Verification items for the finished model (mm, model axes). A direction names the side the tool comes from. Round coordinates to 2 decimals unless told otherwise and drop trailing zeros. Write each loop counter-clockwise with the first axis right and the second up, starting at its lowest first coordinate (ties: lowest second). Pieces come first, ordered by that corner, then holes. Notation, with made-up numbers: M -13.5,-27 L -3.5,-27 A20 cw -3.5,7 Z; hole C 45.5,-27 d6. An arc over 180 degrees is marked long. One line per question, with ' | ' between items. Start each with the question number.
Q1. Cross-section at C-C (y = -2.5). Record the boundary of the cut face in (x, z) (3 decimals).
Q2. Cross-section at B-B (x = -62). Record the boundary of the cut face in (y, z) (3 decimals).
Q3. Tool access check on faces 1 (the face through (92.5, -51.5, -3.9)), 2 (the face through (-99.48, -1, -6)). Record the directions out of +Z, -Z, +X, -X, +Y, -Y that give a thin tool (end or side, any length) a straight path to the whole face; none if there is none.
Q4. Release check for a two-part mould opening along Y. For faces 3 (the face through (94.06, 52.77, -0.74)), 4 (the face through (1, -58.38, -6)), 5 (the face through (-96.172, 55.243, -5.916)) record: released by +Y, released by -Y, zero draft, split by the parting line, or undercut.
Q5. Cross-section at A-A (z = -4). Record the boundary of the cut face in (x, y).
Q6. Thickness scan on line 1 along X through (y, z) = (2.5, -4.25); line 2 along Y through (x, z) = (-22, -3.75); line 3 along Z through (x, y) = (26.5, -16). Record the ranges inside material, lowest first. Write a range as from..to.
Autodesk Inventor part; units mm, degrees
ref_plane "YZ Plane" through (0, 0, 0) normal (1, 0, 0) x (0, 1, 0)
ref_plane "XZ Plane" through (0, 0, 0) normal (0, 1, 0) x (-1, 0, 0)
ref_plane "XY Plane" through (0, 0, 0) normal (0, 0, 1) x (1, 0, 0)
sketch "Sketch1" plane through (0, 0, 0) normal (0, 0, 1) x (1, 0, 0)
  line L0 (77.5, 43.5) -> (77.5, -43.5)
  line L1 (77.5, -43.5) -> (-77.5, -43.5)
  line L2 (-77.5, -43.5) -> (-77.5, 43.5)
  line L3 (-77.5, 43.5) -> (77.5, 43.5)
  line L4 (85.48, 55.38) -> (-85.48, 55.38)
  arc A0 (-85.48, 55.38) -> (-96.48, 44.38) centre (-85.48, 44.38) ccw
  line L5 (-96.48, 44.38) -> (-96.48, -44.38)
  arc A1 (-96.48, -44.38) -> (-85.48, -55.38) centre (-85.48, -44.38) ccw
  line L6 (-85.48, -55.38) -> (85.48, -55.38)
  arc A2 (85.48, -55.38) -> (96.48, -44.38) centre (85.48, -44.38) ccw
  line L7 (96.48, -44.38) -> (96.48, 44.38)
  arc A3 (96.48, 44.38) -> (85.48, 55.38) centre (85.48, 44.38) ccw
  line L8 (-88.48, 58.38) -> (88.48, 58.38)
  line L9 (99.48, 47.38) -> (99.48, -47.38)
  line L10 (88.48, -58.38) -> (-88.48, -58.38)
  line L11 (-99.48, -47.38) -> (-99.48, 47.38)
  arc A4 (-88.48, 58.38) -> (-99.48, 47.38) centre (-88.48, 47.38) ccw
  arc A5 (99.48, 47.38) -> (88.48, 58.38) centre (88.48, 47.38) ccw
  arc A6 (88.48, -58.38) -> (99.48, -47.38) centre (88.48, -47.38) ccw
  arc A7 (-99.48, -47.38) -> (-88.48, -58.38) centre (-88.48, -47.38) ccw
  point P0 (0, 0)
  dimension "d0" = 3
  dimension "d1" = 3
  dimension "d2" = 3
  dimension "d3" = 3
  dimension "d4" = 11
  dimension "d5" = 11
extrude "Extrusion1" add sketch "Sketch1" against normal blind 12 contours L0 L1 L2 L3 | A3 L7 A2 L6 A1 L5 A0 L4 | L8 A5 L9 A6 L10 A7 L11 A4
sketch "Sketch2" plane through (0, 0, 0) normal (0, 0, 1) x (1, 0, 0)
  line L0 (-88.48, 58.38) -> (88.48, 58.38)
  arc A0 (-88.48, 58.38) -> (-99.48, 47.38) centre (-88.48, 47.38) ccw
  line L1 (-99.48, -47.38) -> (-99.48, 47.38)
  arc A1 (-99.48, -47.38) -> (-88.48, -58.38) centre (-88.48, -47.38) ccw
  line L2 (88.48, -58.38) -> (-88.48, -58.38)
  arc A2 (88.48, -58.38) -> (99.48, -47.38) centre (88.48, -47.38) ccw
  line L3 (99.48, 47.38) -> (99.48, -47.38)
  arc A3 (99.48, 47.38) -> (88.48, 58.38) centre (88.48, 47.38) ccw
  line L4 (77.5, 43.5) -> (77.5, -43.5)
  line L5 (77.5, -43.5) -> (-77.5, -43.5)
  line L6 (-77.5, -43.5) -> (-77.5, 43.5)
  line L7 (-77.5, 43.5) -> (77.5, 43.5)
  line L8 (85.48, 55.38) -> (-85.48, 55.38)
  arc A4 (-85.48, 55.38) -> (-96.48, 44.38) centre (-85.48, 44.38) ccw
  line L9 (-96.48, 44.38) -> (-96.48, -44.38)
  arc A5 (-96.48, -44.38) -> (-85.48, -55.38) centre (-85.48, -44.38) ccw
  line L10 (-85.48, -55.38) -> (85.48, -55.38)
  arc A6 (85.48, -55.38) -> (96.48, -44.38) centre (85.48, -44.38) ccw
  line L11 (96.48, -44.38) -> (96.48, 44.38)
  arc A7 (96.48, 44.38) -> (85.48, 55.38) centre (85.48, 44.38) ccw
  arc A8 (-85.48, 56.38) -> (-97.48, 44.38) centre (-85.48, 44.38) ccw
  line L12 (-85.48, 56.38) -> (85.48, 56.38)
  arc A9 (97.48, 44.38) -> (85.48, 56.38) centre (85.48, 44.38) ccw
  line L13 (97.48, 44.38) -> (97.48, -44.38)
  arc A10 (85.48, -56.38) -> (97.48, -44.38) centre (85.48, -44.38) ccw
  line L14 (85.48, -56.38) -> (-85.48, -56.38)
  arc A11 (-97.48, -44.38) -> (-85.48, -56.38) centre (-85.48, -44.38) ccw
  line L15 (-97.48, -44.38) -> (-97.48, 44.38)
  point P0 (0, 0)
  dimension "d8" = 1
extrude "Extrusion2" cut sketch "Sketch2" against normal blind 1.5 contours L4 L5 L6 L7 | A7 L11 A6 L10 A5 L9 A4 L8 | L12 A9 L13 A10 L14 A11 L15 A8
sketch "Sketch3" plane through (0, 0, -1.5) normal (0, 0, 1) x (1, 0, 0)
  arc A0 (-85.48, 56.38) -> (-97.48, 44.38) centre (-85.48, 44.38) ccw
  line L0 (-97.48, -44.38) -> (-97.48, 44.38)
  arc A1 (-97.48, -44.38) -> (-85.48, -56.38) centre (-85.48, -44.38) ccw
  line L1 (85.48, -56.38) -> (-85.48, -56.38)
  arc A2 (85.48, -56.38) -> (97.48, -44.38) centre (85.48, -44.38) ccw
  line L2 (97.48, 44.38) -> (97.48, -44.38)
  arc A3 (97.48, 44.38) -> (85.48, 56.38) centre (85.48, 44.38) ccw
  line L3 (-85.48, 56.38) -> (85.48, 56.38)
  arc A4 (-85.48, 54.38) -> (-95.48, 44.38) centre (-85.48, 44.38) ccw
  line L4 (-85.48, 54.38) -> (85.48, 54.38)
  arc A5 (95.48, 44.38) -> (85.48, 54.38) centre (85.48, 44.38) ccw
  line L5 (95.48, 44.38) -> (95.48, -44.38)
  arc A6 (85.48, -54.38) -> (95.48, -44.38) centre (85.48, -44.38) ccw
  line L6 (85.48, -54.38) -> (-85.48, -54.38)
  arc A7 (-95.48, -44.38) -> (-85.48, -54.38) centre (-85.48, -44.38) ccw
  line L7 (-95.48, -44.38) -> (-95.48, 44.38)
  point P0 (0, 0)
  dimension "d11" = 2
extrude "Extrusion3" cut sketch "Sketch3" against normal blind 8 contours L4 A5 L5 A6 L6 A7 L7 A4
fillet "Fillet1" radius 3.175 8 edges at (92.5511, 51.4511, -9.5) (95.48, 0, -9.5) (92.5511, -51.4511, -9.5) (0, -54.38, -9.5) (-92.5511, -51.4511, -9.5) (-95.48, 0, -9.5) (-92.5511, 51.4511, -9.5) (0, 54.38, -9.5)
sketch "Sketch4" plane through (0, 0, -12) normal (0, 0, -1) x (-1, 0, 0)
  line L0 (-35.15, 31.45) -> (43.7742, 31.45)
  arc A0 (46.7742, 28.45) -> (43.7742, 31.45) centre (43.7742, 28.45) ccw
  line L1 (46.7742, 28.45) -> (46.7742, -21.55)
  arc A1 (43.7742, -24.55) -> (46.7742, -21.55) centre (43.7742, -21.55) ccw
  line L2 (43.7742, -24.55) -> (-35.15, -24.55)
  arc A2 (-38.15, -21.55) -> (-35.15, -24.55) centre (-35.15, -21.55) ccw
  line L3 (-38.15, -21.55) -> (-38.15, 28.45)
  arc A3 (-35.15, 31.45) -> (-38.15, 28.45) centre (-35.15, 28.45) ccw
  line L4 (-48.26, 38.1) -> (48.26, 38.1)
  line L5 (50.8, 35.56) -> (50.8, -35.56)
  line L6 (48.26, -38.1) -> (-48.26, -38.1)
  line L7 (-50.8, -35.56) -> (-50.8, 35.56)
  arc A4 (-48.26, 38.1) -> (-50.8, 35.56) centre (-48.26, 35.56) ccw
  arc A5 (50.8, 35.56) -> (48.26, 38.1) centre (48.26, 35.56) ccw
  arc A6 (48.26, -38.1) -> (50.8, -35.56) centre (48.26, -35.56) ccw
  arc A7 (-50.8, -35.56) -> (-48.26, -38.1) centre (-48.26, -35.56) ccw
  point P0 (0, 0)
  point P1 (-50.8, 38.1)
  point P2 (50.8, 38.1)
  point P3 (-50.8, -38.1)
  dimension "d15" = 101.6
  dimension "d16" = 76.2
  dimension "d17" = 38.1
  dimension "d18" = 50.8
  dimension "d19" = 2.54
equation "\"d1\" = d0"
equation "\"d2\" = d0"
equation "\"d3\" = d0"
equation "\"d4\" = d5"
properties part number "Hub Enclosure"
Determined:
1) outline: M -99.48,-12 L 99.48,-12 L 99.48,0 L 97.48,0 L 97.48,-1.5 L 95.48,-1.5 L 95.48,-6.325 A3.175 cw 92.305,-9.5 L -92.305,-9.5 A3.175 cw -95.48,-6.325 L -95.48,-1.5 L -97.48,-1.5 L -97.48,0 L -99.48,0 Z
2) outline: M -58.38,-12 L 58.38,-12 L 58.38,0 L 56.38,0 L 56.38,-1.5 L 54.38,-1.5 L 54.38,-6.325 A3.175 cw 51.205,-9.5 L -51.205,-9.5 A3.175 cw -54.38,-6.325 L -54.38,-1.5 L -56.38,-1.5 L -56.38,0 L -58.38,0 Z
3) face 1: +Z | face 2: +Z, -Z, -X, +Y, -Y
4) face 3: undercut | face 4: released by -Y | face 5: released by +Y
5) outline: M -99.48,-47.38 A11 ccw -88.48,-58.38 L 88.48,-58.38 A11 ccw 99.48,-47.38 L 99.48,47.38 A11 ccw 88.48,58.38 L -88.48,58.38 A11 ccw -99.48,47.38 Z; hole M -95.48,-44.38 A10 ccw -85.48,-54.38 L 85.48,-54.38 A10 ccw 95.48,-44.38 L 95.48,44.38 A10 ccw 85.48,54.38 L -85.48,54.38 A10 ccw -95.48,44.38 Z
6) line 1: x = -99.48..-95.48, 95.48..99.48 | line 2: y = -58.38..-54.38, 54.38..58.38 | line 3: z = -12..-9.5
